Drawing for the job (mm, zero at the part's lowest x, y, z). A direction names the side the tool comes from. Coordinates: 2 decimals unless noted, no trailing zeros. Write each loop counter-clockwise with the first axis right and the second up, starting at its lowest first coordinate (ties: lowest second). Pieces come first, ordered by that corner, then holes. Notation, with made-up numbers: M 34,89 L 92,89 A20 ccw 92,98 Z; hole C 67,-18.5 d5. An arc over 180 degrees is marked long. Put each result on its own line as item: value. Start each with the question number.
Q1. Cut at D-D (x = 82). Write the cut outline in (y, z), then the cut area to 3 significant figures.
Q2. Cut at C-C (x = 52). Write the cut outline in (y, z).
Q3. Cut at B-B (y = 20.25). Write the cut outline in (x, z) (3 decimals), then the cut area to 3 significant figures.
Q4. Drill centre lines: line 1 along X through (y, z) = (18.75, 13); line 2 along X through (y, z) = (4.75, 86); line 3 along X through (y, z) = (10.75, 62). Where is each one in solid material? Low to high.
Q5. Which spindle directions (+Z, -Z, +X, -X, +Y, -Y) get a long thin tool onto all of the face, cutting with end or side? Do the marked faces 5, 6 and 7. Say none if no direction does.
Q6. Cut at A-A (z = 65). Write the cut outline in (x, y).
Q7. Pull direction X, two halves, no side cores. Call the marked faces 1, 2, 3 and 4: pulls with the +X half, pulls with the -X half, needs draft (parallel to the pull), parting line crosses it, or undercut.
Q8. Drop flat-ended pins along their axis: pin 1 (10 mm diameter, centred on y = 3, z = 40.5, fed in from +X); pin 2 (12.5 mm diameter, centred on x = 26.5, y = 11, fed in from -Z); pin 3 (7 mm diameter, centred on y = 15.5, z = 17, fed in from -X). Give the stop position or say it passes through.
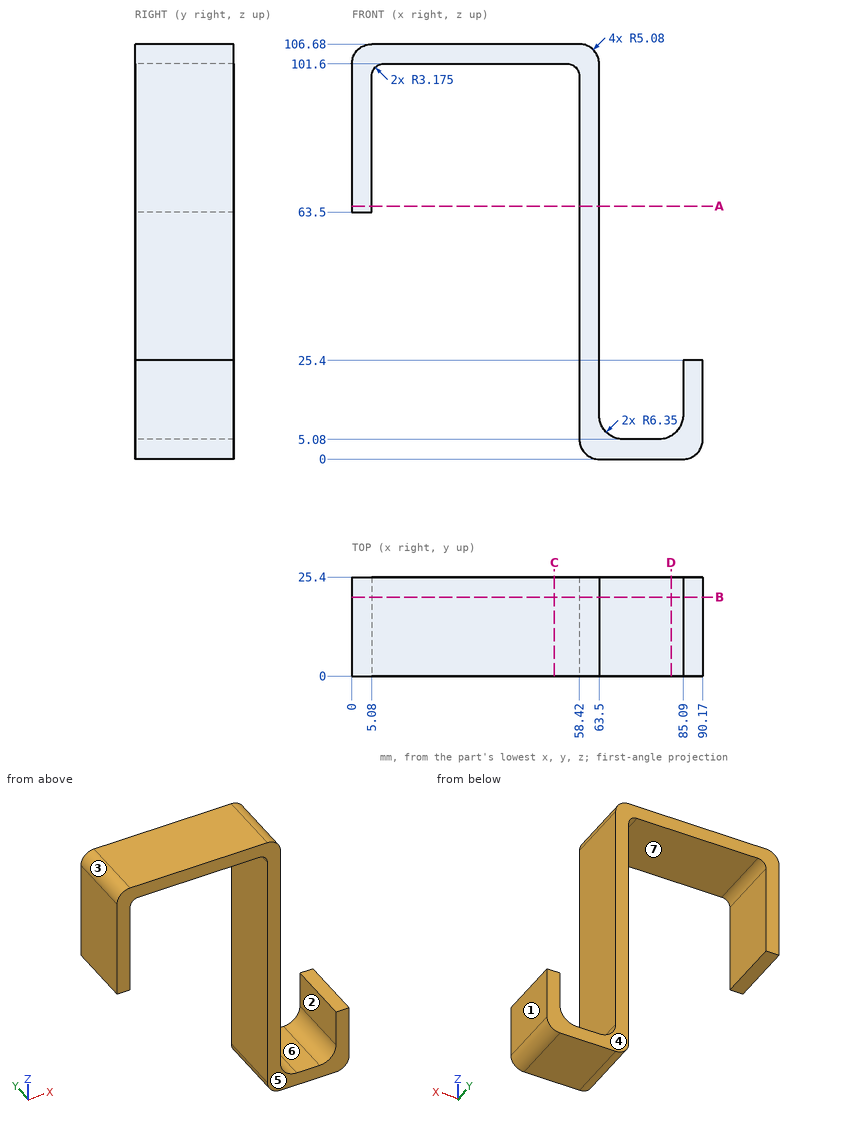
Computed values:
1. outline: M 0,0 L 25.4,0 L 25.4,5.98 L 0,5.98 Z
1. area: 152 mm2
2. outline: M 0,101.6 L 25.4,101.6 L 25.4,106.68 L 0,106.68 Z
3. outline: M 0,63.5 L 5.08,63.5 L 5.08,98.425 A3.175 cw 8.255,101.6 L 55.245,101.6 A3.175 cw 58.42,98.425 L 58.42,5.08 A5.08 ccw 63.5,0 L 85.09,0 A5.08 ccw 90.17,5.08 L 90.17,25.4 L 85.09,25.4 L 85.09,11.43 A6.35 cw 78.74,5.08 L 69.85,5.08 A6.35 cw 63.5,11.43 L 63.5,101.6 A5.08 ccw 58.42,106.68 L 5.08,106.68 A5.08 ccw 0,101.6 Z
3. area: 1,270 mm2
4. line 1: 58.42 to 63.5, 85.09 to 90.17
4. line 2: 0 to 5.08, 58.42 to 63.5
4. line 3: 58.42 to 63.5
5. face 5: +Z, -Z, +X, -X, -Y
5. face 6: +Z, +Y, -Y
5. face 7: -Z, +Y, -Y
6. outline: M 0,0 L 5.08,0 L 5.08,25.4 L 0,25.4 Z; M 58.42,0 L 63.5,0 L 63.5,25.4 L 58.42,25.4 Z
7. face 1: pulls with the +X half
7. face 2: undercut
7. face 3: pulls with the -X half
7. face 4: needs draft
8. pin 1: x = 63.5
8. pin 2: z = 101.6
8. pin 3: x = 58.42
